Answer from the drawing. Dimensions are ordinates in mm from the lowest x, y and z of the part. Round coordinates to 2 decimals unless told otherwise and drop trailing zeros. Write each loop counter-clockwise with the first axis right and the second up, starting at its lowest first coordinate (ties: lowest second). Pieces come first, ordered by that corner, then holes. Notation, with made-up numbers: (-33.5, -17) - (8.5, -17) arc R21 ccw to (8.5, 0) - close; hole circle Ø7 at (-18, 60.25). An arc over 180 degrees is marked (long way). Answer as a JSON object with one key per item and string values.
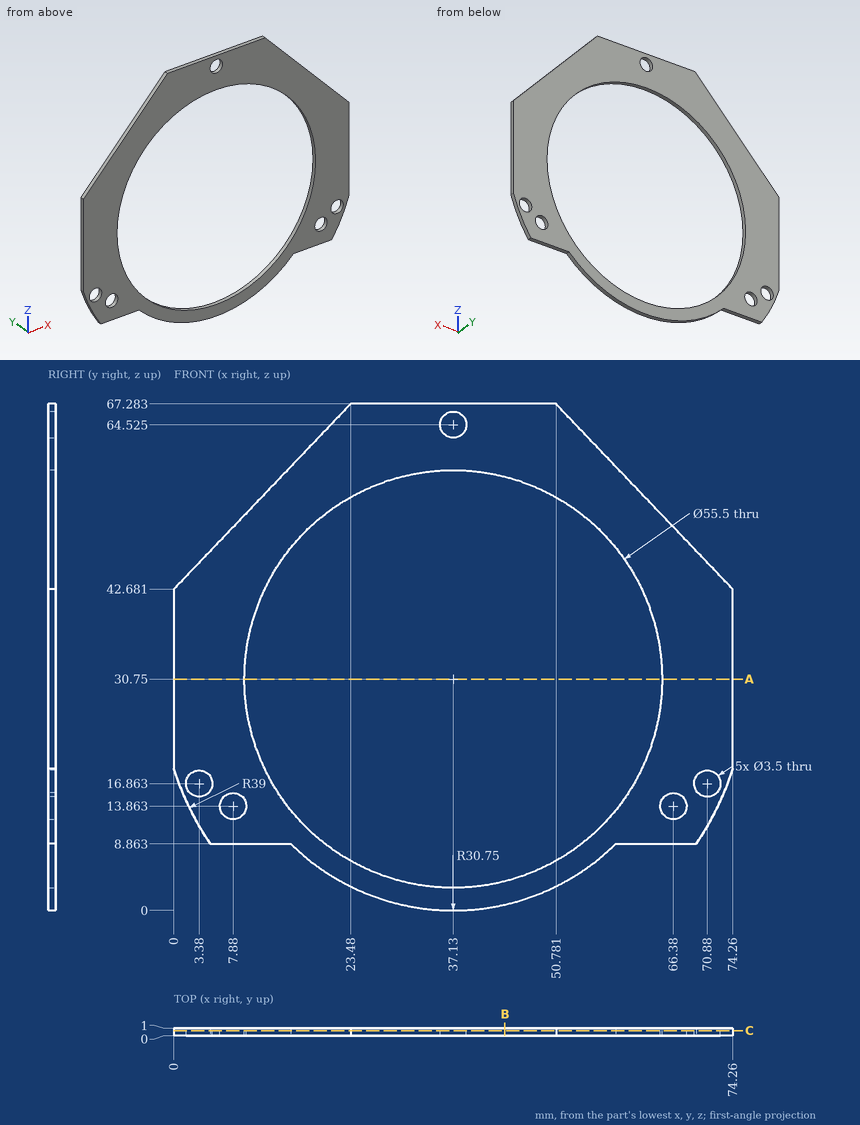
Item 1: Consider line 1 along X through (y, z) = (0.7, 30.75); line 2 along X through (y, z) = (0.8, 17) (1 decimal); line 3 along Z through (x, y) = (58, 0.1) (1 decimal). Determine where each line is inside the solid, lowest interval first.
Results found:
{"line 1": "0 to 9.38, 64.88 to 74.26", "line 2": "0.6 to 1.6, 5.1 to 13, 61.2 to 69.1, 72.6 to 73.6", "line 3": "8.2 to 12.5, 49 to 59.7"}
Item 2: This flat-tipped pin is pushed along its axis until it touches: P1, Ø2, axis at x = 37.13, z = 64.52, coming from the +Y side. Where does it stop, or does it pass through?
Results found:
{"P1": "through"}
Item 3: A cutting plane is placed at B-B (x = 44). Write down the section's boundary in (y, z).
Results found:
{"outline": "(0, 0.78) - (1, 0.78) - (1, 3.86) - (0, 3.86) - close; (0, 57.64) - (1, 57.64) - (1, 67.28) - (0, 67.28) - close"}
Item 4: A cutting plane is placed at C-C (y = 0.7). Give the number of separate pieces and of enclosed holes in the cut face, and give its area (3 significant figures).
Results found:
{"separate pieces": "1", "enclosed holes": "6", "area": "1,510 mm²"}
Item 5: A cutting plane is placed at A-A (z = 30.75). Write down the section's boundary in (x, y).
Results found:
{"outline": "(0, 0) - (9.38, 0) - (9.38, 1) - (0, 1) - close; (64.88, 0) - (74.26, 0) - (74.26, 1) - (64.88, 1) - close"}
